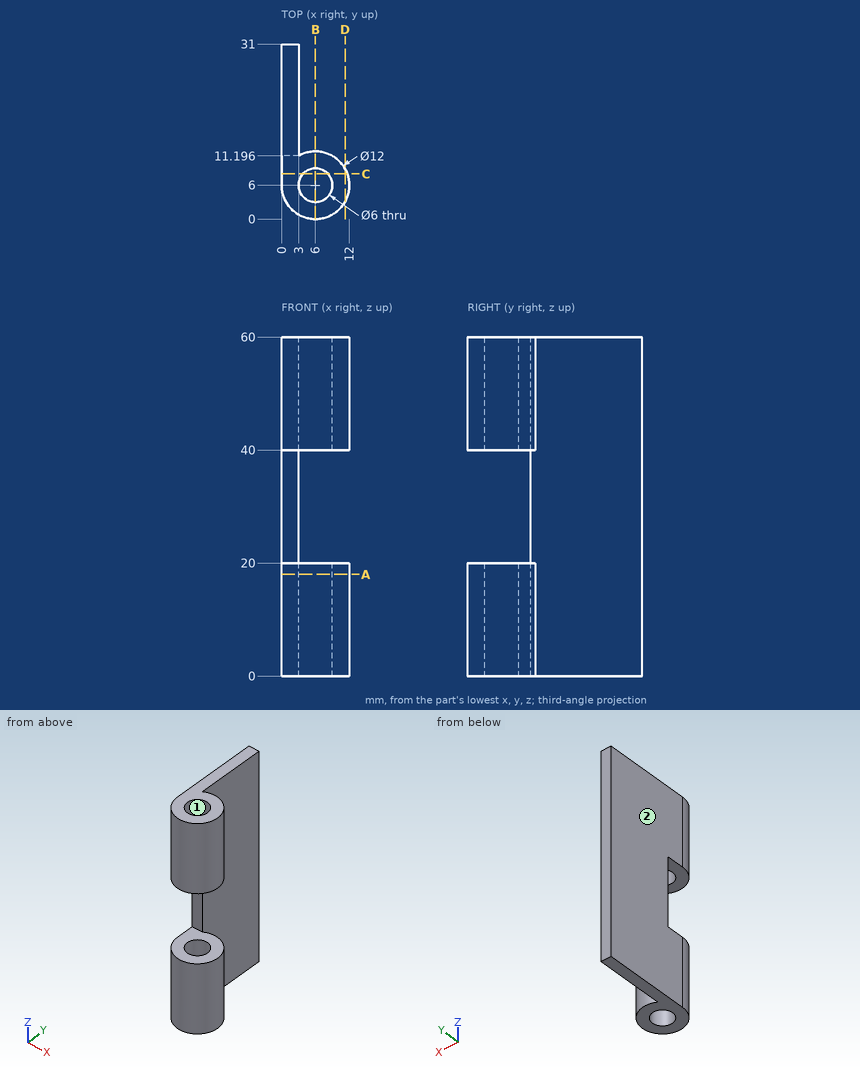
For this review, use the dimensioned drawing (mm, ordinates from the lowest corner) and the shaded views. Round coordinates to 2 decimals unless told otherwise and drop trailing zeros. Write each loop counter-clockwise with the first axis right and the second up, starting at its lowest first coordinate (ties: lowest second). Pieces come first, ordered by that corner, then holes. Notation, with made-up numbers: (-38.5, 50) - (-4.5, 50) arc R13 cw to (-4.5, 59) - close; hole circle Ø1 at (-14.75, 24). An arc over 180 degrees is marked (long way). Use a Markdown table: item, result.
Q1. Clearance check with flat-ended pins moving along their axes: pin 1 (5 mm diameter, centred on x = 6, y = 6, fed in from -Z); pin 2 (1 mm diameter, centred on x = 7.5, z = 11.5, fed in from -Y); pin 3 (2.5 mm diameter, centred on x = 1.5, z = 30.5, fed in from -Y); pin 4 (6 mm diameter, centred on y = 24, z = 21.5, fed in from +X). State where each tip first meets the part, or that it passes through.
Derived:
| item | result |
|---|---|
| pin 1 | passes through |
| pin 2 | stops at y = 0.08 |
| pin 3 | stops at y = 11.2 |
| pin 4 | stops at x = 3 |
Q2. We need section B-B (x = 6). Give the boundary of the cut face in (y, z).
Derived:
| item | result |
|---|---|
| outline | (0, 0) - (3, 0) - (3, 20) - (0, 20) - close; (0, 40) - (3, 40) - (3, 60) - (0, 60) - close; (9, 0) - (12, 0) - (12, 20) - (9, 20) - close; (9, 40) - (12, 40) - (12, 60) - (9, 60) - close |
Q3. Wall thickness on line 1 along Z through (x, y) = (2, 4); line 2 along Y through (x, z) = (6, 44); line 3 along Y through (x, z) = (4, 55): over which ranges is each line inside the solid? List them lowest first.
Derived:
| item | result |
|---|---|
| line 1 | z = 0 to 20, 40 to 60 |
| line 2 | y = 0 to 3, 9 to 12 |
| line 3 | y = 0.34 to 3.76, 8.24 to 11.66 |
Q4. We need section A-A (z = 18). Give the boundary of the cut face in (x, y).
Derived:
| item | result |
|---|---|
| outline | (0, 6) arc R6 ccw (long way) to (3, 11.2) - (3, 31) - (0, 31) - close; hole circle Ø6 at (6, 6) |
Q5. We need section D-D (x = 11.25). Give the boundary of the cut face in (y, z) (1 decimal).
Derived:
| item | result |
|---|---|
| outline | (3.1, 0) - (8.9, 0) - (8.9, 20) - (3.1, 20) - close; (3.1, 40) - (8.9, 40) - (8.9, 60) - (3.1, 60) - close |
Q6. We need section C-C (y = 8). Give the boundary of the cut face in (x, z), plus the area to 3 significant figures.
Derived:
| item | result |
|---|---|
| outline | (0, 0) - (3.76, 0) - (3.76, 20) - (0, 20) - close; (0, 40) - (3.76, 40) - (3.76, 60) - (0, 60) - close; (8.24, 0) - (11.66, 0) - (11.66, 20) - (8.24, 20) - close; (8.24, 40) - (11.66, 40) - (11.66, 60) - (8.24, 60) - close |
| area | 287 mm2 |
Q7. The part is to be moulded in two halves that separate along X. For the marked faces 1 and 2, say which applies: pulls with the +X half, pulls with the -X half, needs draft (parallel to the pull), parting line crosses it, or undercut.
Derived:
| item | result |
|---|---|
| face 1 | undercut |
| face 2 | pulls with the -X half |
